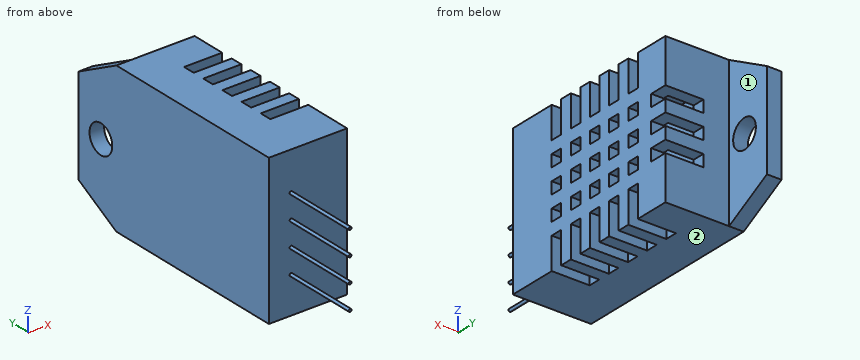
from build123d import *

# Parameters (mm, degrees)
SKETCH1_W           = 15.47
SKETCH1_H           = 20.15
BOSS_EXTRUDE1_DEPTH = 8.15
SKETCH1_4_R         = 1.5
SKETCH1_4_W         = 15.47
SKETCH1_4_H         = 20.15
BOSS_EXTRUDE2_DEPTH = 1.52
SHELL1_START        = -6.455
SHELL1_OUTLINE_W    = 5.59
SHELL1_OUTLINE_H    = 17.59
SHELL1_DEPTH        = 12.91
SKETCH2_W           = 1.25
SKETCH2_H           = 1.87
SKETCH2_H_2         = 1.264229858
SKETCH2_W_2         = 3.3
CUT_EXTRUDE1_DEPTH  = 3.96
SKETCH3_R           = 0.15
BOSS_EXTRUDE3_DEPTH = 7.8


# Read off the part's stored shape, not the designer's step: Shell1
with BuildPart() as part:
    # Sketch1 → Boss-Extrude1 (new body)
    with BuildSketch(Plane(origin=(0, 0, 0), x_dir=(0, 0, -1), z_dir=(1, 0, 0))):
        with Locations((0, -2.5)):
            Rectangle(SKETCH1_W, SKETCH1_H)
    extrude(amount=BOSS_EXTRUDE1_DEPTH)

    # Sketch1<4> → Boss-Extrude2 (add)
    # profile 1 of 2: a face of its own
    with BuildSketch(Plane(origin=(0, 0, 0), x_dir=(0, 0, -1), z_dir=(1, 0, 0))):
        Polygon((-5.035, 12.575), (-7.735, 7.575), (7.735, 7.575), (5.035, 12.575), align=None)
        with Locations((0, 9.615)):
            Circle(SKETCH1_4_R, mode=Mode.SUBTRACT)
    # profile 2 of 2: a face of its own
    with BuildSketch(Plane(origin=(0, 0, 0), x_dir=(0, 0, -1), z_dir=(1, 0, 0))):
        with Locations((0, -2.5)):
            Rectangle(SKETCH1_4_W, SKETCH1_4_H)
    extrude(amount=BOSS_EXTRUDE2_DEPTH)

    # Shell1 outline → Shell1 (cut)
    with BuildSketch(Plane.XY.offset(SHELL1_START)):
        with Locations((4.075, -2.5)):
            Rectangle(SHELL1_OUTLINE_W, SHELL1_OUTLINE_H)
    extrude(amount=SHELL1_DEPTH, mode=Mode.SUBTRACT)

    # Sketch2 → Cut-Extrude1 (cut)
    with BuildSketch(Plane(origin=(8.15, 0, 0), x_dir=(0, 0, -1), z_dir=(1, 0, 0))):
        with Locations((0, 6.64)):
            Rectangle(SKETCH2_W, SKETCH2_H)
        with Locations((2.53, 6.64)):
            Rectangle(SKETCH2_W, SKETCH2_H)
        with Locations((2.53, 0.772885071)):
            Rectangle(SKETCH2_W, SKETCH2_H_2)
        with Locations((6.085, 0.772885071)):
            Rectangle(SKETCH2_W_2, SKETCH2_H_2)
        with Locations((6.085, 3.302885071)):
            Rectangle(SKETCH2_W_2, SKETCH2_H_2)
        with Locations((0, 3.302885071)):
            Rectangle(SKETCH2_W, SKETCH2_H_2)
        with Locations((-2.53, 0.772885071)):
            Rectangle(SKETCH2_W, SKETCH2_H_2)
        with Locations((-2.53, 3.302885071)):
            Rectangle(SKETCH2_W, SKETCH2_H_2)
        with Locations((-6.085, 3.302885071)):
            Rectangle(SKETCH2_W_2, SKETCH2_H_2)
        with Locations((-6.085, 0.772885071)):
            Rectangle(SKETCH2_W_2, SKETCH2_H_2)
        with Locations((-6.085, -1.757114929)):
            Rectangle(SKETCH2_W_2, SKETCH2_H_2)
        with Locations((-6.085, -4.287114929)):
            Rectangle(SKETCH2_W_2, SKETCH2_H_2)
        with Locations((-2.53, -1.757114929)):
            Rectangle(SKETCH2_W, SKETCH2_H_2)
        with Locations((0, -1.757114929)):
            Rectangle(SKETCH2_W, SKETCH2_H_2)
        with Locations((2.53, -1.757114929)):
            Rectangle(SKETCH2_W, SKETCH2_H_2)
        with Locations((6.085, -1.757114929)):
            Rectangle(SKETCH2_W_2, SKETCH2_H_2)
        with Locations((6.085, -4.287114929)):
            Rectangle(SKETCH2_W_2, SKETCH2_H_2)
        with Locations((2.53, -4.287114929)):
            Rectangle(SKETCH2_W, SKETCH2_H_2)
        with Locations((0, -4.287114929)):
            Rectangle(SKETCH2_W, SKETCH2_H_2)
        with Locations((-2.53, -4.287114929)):
            Rectangle(SKETCH2_W, SKETCH2_H_2)
        with Locations((6.085, -6.817114929)):
            Rectangle(SKETCH2_W_2, SKETCH2_H_2)
        with Locations((2.53, -6.817114929)):
            Rectangle(SKETCH2_W, SKETCH2_H_2)
        with Locations((-2.53, -6.817114929)):
            Rectangle(SKETCH2_W, SKETCH2_H_2)
        with Locations((-6.085, -6.817114929)):
            Rectangle(SKETCH2_W_2, SKETCH2_H_2)
        with Locations((-2.53, 6.64)):
            Rectangle(SKETCH2_W, SKETCH2_H)
        with Locations((2.53, 3.302885071)):
            Rectangle(SKETCH2_W, SKETCH2_H_2)
        with Locations((0, 0.772885071)):
            Rectangle(SKETCH2_W, SKETCH2_H_2)
        with Locations((0, -6.817114929)):
            Rectangle(SKETCH2_W, SKETCH2_H_2)
    extrude(amount=-CUT_EXTRUDE1_DEPTH, mode=Mode.SUBTRACT)

    # Sketch3 → Boss-Extrude3 (add)
    with BuildSketch(Plane.XZ.offset(12.575)):
        with Locations(Location((2.31, 3.704312159, 0), (0, 0, 90))):
            Circle(SKETCH3_R)
        with Locations(Location((2.31, 1.164312159, 0), (0, 0, 90))):
            Circle(SKETCH3_R)
        with Locations(Location((2.31, -1.375687841, 0), (0, 0, 90))):
            Circle(SKETCH3_R)
        with Locations(Location((2.31, -3.915687841, 0), (0, 0, 90))):
            Circle(SKETCH3_R)
    extrude(amount=BOSS_EXTRUDE3_DEPTH)


solid = part.part
Could you check a few things on this model? Use its own coordinates, in mm. Face numbers are marked on the shaded views. A direction names the side the tool comes from. Give positions to 0.01 mm unless a question says otherwise; leave off trailing zeros. Order: outer loops, then holes, each group sorted by start corner. A loop starts at its lowest first (then second) coordinate and runs counter-clockwise, first axis right, second up. Notation, with made-up numbers: (-10.5, 16.25) -> (15.5, 16.25) arc R10 cw to (15.5, 31.25) -> close; hole circle Ø11 at (5.25, 23.25). An arc over 180 degrees is marked (long way). Answer in a Markdown table with one row per item. Add a question column.
Item 1: I'm going to push flat-ended pins straight in: P1, Ø3.5, axis at x = 7, z = 6.5, coming from the +Y side (3 decimals); P2, Ø0.6, axis at x = 7.5, z = 2.5, coming from the -Y side (3 decimals); P3, Ø0.6, axis at x = 7.5, y = 3.5, coming from the -Z side (3 decimals). Where does each tip first touch, or does it pass through?
Item 2: Imagine slicing it at B-B (x = 3.25). List the corners of the cut face in (y, z) for me (3 decimals).
Item 3: For the marked faces 1 and 2, which set-ups out of +Z, -Z, +X, -X, +Y, -Y let a thin tool reach every point of the face, with its end or its side?
Item 4: Imagine slicing it at C-C (z = 5.75). Count the separate pieces of the cut face and the enclosed holes in it, and give its area (3 significant figures).
Item 5: Imagine slicing it at A-A (y = -2). List the corners of the cut face in (x, z) for me (3 decimals), and give its area (3 significant figures).
Item 6: Please list where these lines run through material, in increasing order: probe 1 along Z at (x, y) = (6.5, 6.5) (3 decimals); probe 2 along Z at (x, y) = (2.5, -5.5) (3 decimals); probe 3 along Y at (x, z) = (4.5, -1) (3 decimals).
Result:
| question | item | result |
|---|---|---|
| 1 | P1 | y = 7.575 |
| 1 | P2 | y = -12.575 |
| 1 | P3 | z = -4.435 |
| 2 | outline | (-12.575, -7.735) -> (7.575, -7.735) -> (7.575, 7.735) -> (-12.575, 7.735) -> close; hole (-11.295, -6.455) -> (6.295, -6.455) -> (6.295, 6.455) -> (-11.295, 6.455) -> close |
| 3 | face 1 | +Z, -Z, +X, +Y |
| 3 | face 2 | -Z, +X, -X, +Y, -Y |
| 4 | separate pieces | 5 |
| 4 | enclosed holes | 0 |
| 4 | area | 63.4 mm2 |
| 5 | outline | (0, -7.735) -> (4.19, -7.735) -> (4.19, -6.455) -> (1.28, -6.455) -> (1.28, 6.455) -> (4.19, 6.455) -> (4.19, 7.735) -> (0, 7.735) -> close; (6.87, -4.435) -> (8.15, -4.435) -> (8.15, -3.155) -> (6.87, -3.155) -> close; (6.87, -1.905) -> (8.15, -1.905) -> (8.15, -0.625) -> (6.87, -0.625) -> close; (6.87, 0.625) -> (8.15, 0.625) -> (8.15, 1.905) -> (6.87, 1.905) -> close; (6.87, 3.155) -> (8.15, 3.155) -> (8.15, 4.435) -> (6.87, 4.435) -> close |
| 5 | area | 33.8 mm2 |
| 6 | probe 1 | -7.735 to -3.155, -1.905 to -0.625, 0.625 to 1.905, 3.155 to 7.735 |
| 6 | probe 2 | -7.735 to -6.455, 6.455 to 7.735 |
| 6 | probe 3 | -12.575 to -11.295, 6.295 to 7.575 |
